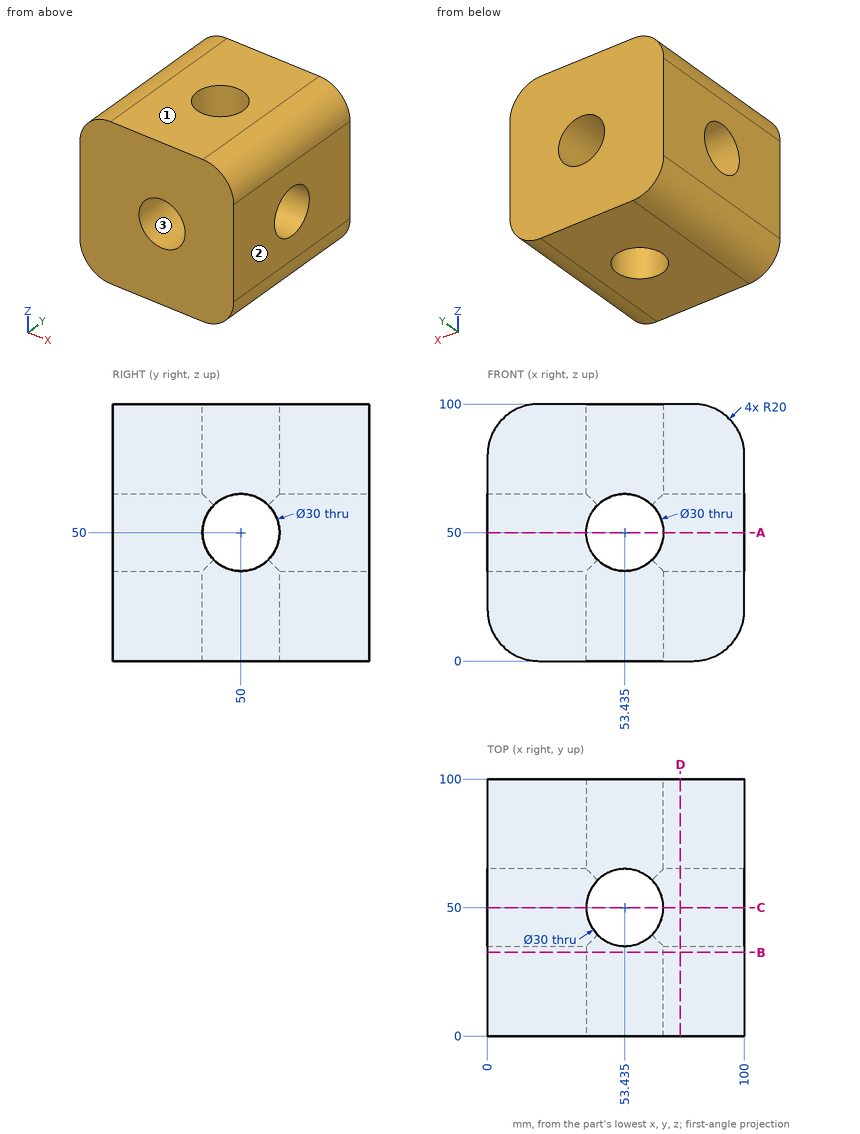
Check sheet for the drawn part. Datum: minimum x, y, z corner. Units: mm. Round coordinates to 2 decimals unless told otherwise and drop trailing zeros. Loops run counter-clockwise (first coordinate to the right, second up) from the corner with the lowest first, then second, coordinate; pieces in that order, holes last. Notation, with made-up numbers: (39, 40) -> (50, 40) arc R10 cw to (50, 57) -> close; hole circle Ø11 at (60, -21). An arc over 180 degrees is marked (long way). Put each result on its own line as item: value. Start each with the question number.
1. Scan lines: probe 1 along X at (y, z) = (50, 77) (3 decimals); probe 2 along Y at (x, z) = (13.5, 53.5); probe 3 along Y at (x, z) = (43, 90.5) (1 decimal). Record each from-to range of solid material in increasing order.
2. Section check D-D (x = 75). Enter the section's corners in (y, z), plus the area to 3 significant figures.
3. Draft check along Z on the marked faces 1, 2 and 3. Enter one of: +Z half, -Z half, draft (parallel to the pull), parting line (faces both ways), or undercut.
4. Section check C-C (y = 50). Enter the section's corners in (x, z) (3 decimals), plus the area to 3 significant figures.
5. Section check A-A (z = 50). Enter the section's corners in (x, y) (3 decimals), plus the area to 3 significant figures.
6. Gauge pin test, flat ends, axial feed: pin 1 (1 mm diameter, centred on x = 59, z = 30, fed in from -Y); pin 2 (12 mm diameter, centred on x = 13.5, y = 15.5, fed in from -Z). Record the tip position at first contact, or that the pin passes through.
7. Section check B-B (y = 32.5). Enter the section's corners in (x, z) (3 decimals).
Findings:
1. probe 1: x = 0 to 38.435, 68.435 to 100
1. probe 2: y = 0 to 35.41, 64.59 to 100
1. probe 3: y = 0 to 39.2, 60.8 to 100
2. outline: (0, 0) -> (100, 0) -> (100, 100) -> (0, 100) -> close; hole circle Ø30 at (50, 50)
2. area: 9,290 mm^2
3. face 1: +Z half
3. face 2: draft
3. face 3: undercut
4. outline: (0, 20) arc R20 ccw to (20, 0) -> (38.435, 0) -> (38.435, 35) -> (0, 35) -> close; (0, 65) -> (38.435, 65) -> (38.435, 100) -> (20, 100) arc R20 ccw to (0, 80) -> close; (68.435, 0) -> (80, 0) arc R20 ccw to (100, 20) -> (100, 35) -> (68.435, 35) -> close; (68.435, 65) -> (100, 65) -> (100, 80) arc R20 ccw to (80, 100) -> (68.435, 100) -> close
4. area: 4,560 mm^2
5. outline: (0, 0) -> (38.435, 0) -> (38.435, 35) -> (0, 35) -> close; (0, 65) -> (38.435, 65) -> (38.435, 100) -> (0, 100) -> close; (68.435, 0) -> (100, 0) -> (100, 35) -> (68.435, 35) -> close; (68.435, 65) -> (100, 65) -> (100, 100) -> (68.435, 100) -> close
5. area: 4,900 mm^2
6. pin 1: stops at y = 0
6. pin 2: stops at z = 0.01
7. outline: (0, 20) arc R20 ccw to (20, 0) -> (80, 0) arc R20 ccw to (100, 20) -> (100, 80) arc R20 ccw to (80, 100) -> (20, 100) arc R20 ccw to (0, 80) -> close; hole circle Ø30 at (53.435, 50)
